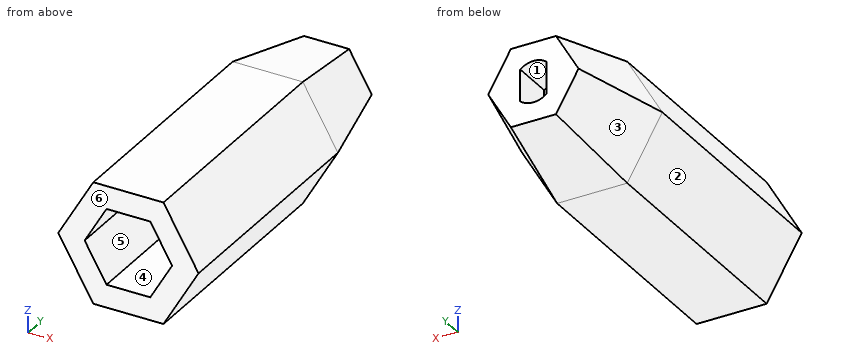
Autodesk Inventor part; units mm, degrees
ref_plane "YZ Plane" through (0, 0, 0) normal (1, 0, 0) x (0, 1, 0)
ref_plane "XZ Plane" through (0, 0, 0) normal (0, 1, 0) x (-1, 0, 0)
ref_plane "XY Plane" through (0, 0, 0) normal (0, 0, 1) x (1, 0, 0)
sketch "Boceto1" plane through (0, 0, 0) normal (0, 1, 0) x (-1, 0, 0)
  line L0 (0, 0) -> (5.8, 0)
  line L1 (5.8, 0) -> (9.3, 0)
  line L2 (5.8, 0) -> (2.9, -5.0229)
  line L3 (2.9, -5.0229) -> (-2.9, -5.0229)
  line L4 (-2.9, -5.0229) -> (-5.8, 0)
  line L5 (-5.8, 0) -> (-2.9, 5.0229)
  line L6 (-2.9, 5.0229) -> (2.9, 5.0229)
  line L7 (2.9, 5.0229) -> (5.8, 0)
  line L8 (9.3, 0) -> (4.65, -8.054)
  line L9 (4.65, -8.054) -> (-4.65, -8.054)
  line L10 (-4.65, -8.054) -> (-9.3, 0)
  line L11 (-9.3, 0) -> (-4.65, 8.054)
  line L12 (-4.65, 8.054) -> (4.65, 8.054)
  line L13 (4.65, 8.054) -> (9.3, 0)
  dimension "d0" = 5.8
  dimension "d1" = 3.5
extrude "Extrusión1" add sketch "Boceto1" along normal blind 30
sketch "Boceto2" plane through (0, 30, 0) normal (0, 1, 0) x (1, 0, 0)
  line L0 (-4.65, 8.054) -> (-9.3, 0)
  line L1 (-9.3, 0) -> (-4.65, 8.054)
  line L2 (-4.65, 8.054) -> (4.65, 8.054)
  line L3 (4.65, 8.054) -> (9.3, 0)
  line L4 (9.3, 0) -> (4.65, -8.054)
  line L5 (4.65, -8.054) -> (-4.65, -8.054)
  line L6 (-4.65, -8.054) -> (-9.3, 0)
  point P0 (0, 0)
  point P1 (0, 0)
extrude "Extrusión2" add sketch "Boceto2" along normal blind 13.5 draft -12
sketch "Boceto3" plane through (0, 0, 0) normal (0, -1, 0) x (1, 0, 0)
  line L0 (9.3, 0) -> (5.9866, 0)
  line L1 (9.3, 0) -> (4.65, -8.054)
  line L2 (4.65, -8.054) -> (-4.65, -8.054)
  line L3 (-4.65, -8.054) -> (-9.3, 0)
  line L4 (-9.3, 0) -> (-4.65, 8.054)
  line L5 (-4.65, 8.054) -> (4.65, 8.054)
  line L6 (4.65, 8.054) -> (9.3, 0)
  point P0 (0, 0)
  point P1 (0, 0)
sketch "Boceto4" plane through (0, 0, 0) normal (0, -1, 0) x (1, 0, 0)
  line L0 (5.8, 0) -> (2.9, -5.0229)
  line L1 (2.9, -5.0229) -> (-2.9, -5.0229)
  line L2 (-2.9, -5.0229) -> (-5.8, 0)
  line L3 (-5.8, 0) -> (-2.9, 5.0229)
  line L4 (-2.9, 5.0229) -> (2.9, 5.0229)
  line L5 (2.9, 5.0229) -> (5.8, 0)
  point P0 (0, 0)
  point P1 (0, 0)
extrude "Extrusión3" add sketch "Boceto3" along normal blind 2
sketch "Boceto5" plane through (0, -2, 0) normal (0, -1, 0) x (1, 0, 0)
  line L0 (0, 0) -> (5.8, 0)
  line L1 (5.8, 0) -> (2.9, -5.0229)
  line L2 (2.9, -5.0229) -> (-2.9, -5.0229)
  line L3 (-2.9, -5.0229) -> (-5.8, 0)
  line L4 (-5.8, 0) -> (-2.9, 5.0229)
  line L5 (-2.9, 5.0229) -> (2.9, 5.0229)
  line L6 (2.9, 5.0229) -> (5.8, 0)
  dimension "d8" = 5.8
extrude "Extrusión4" cut sketch "Boceto5" against normal blind 2
sketch "Boceto6" plane through (0, 43.5, 0) normal (0, 1, 0) x (1, 0, 0)
  line L0 (-1.75, 0) -> (-1.75, 2.1213)
  line L1 (-1.75, 0) -> (-1.75, -2.1213)
  line L2 (1.75, 0) -> (1.75, 2.1213)
  line L3 (1.75, 0) -> (1.75, -2.1213)
  arc A0 (-1.75, -2.1213) -> (1.75, -2.1213) centre (0, 0) ccw
  arc A1 (1.75, 2.1213) -> (-1.75, 2.1213) centre (0, 0) ccw
extrude "Extrusión5" cut sketch "Boceto6" against normal blind 5.5
properties part number "acopladorV3"
Design review of the part built by this model. Coordinates are the model's own, in mm. Face numbers are marked on the shaded views. A direction names the side the tool comes from. Round coordinates to 2 decimals unless told otherwise and drop trailing zeros. Write each loop counter-clockwise with the first axis right and the second up, starting at its lowest first coordinate (ties: lowest second). Pieces come first, ordered by that corner, then holes. Notation, with made-up numbers: (-32.75, -4) -> (11.25, -4) arc R30 ccw to (11.25, 18) -> close; hole circle Ø8 at (-32, 22.5). An arc over 180 degrees is marked (long way). Write item = value, one per line. Start each with the question number.
1) Wall thickness on probe 1 along Z at (x, y) = (-2, 0); probe 2 along X at (y, z) = (4.5, -0.5); probe 3 along Y at (x, z) = (0.75, -1.25): over which ranges is each line inside the solid? List them lowest first. Write a range as from..to.
2) Take a section at D-D, the plane x = 3.75. State the section outline as (y, z) points.
3) Take a section at C-C, the plane z = 1.25. State the section outline as (x, y) points.
4) Take a section at B-B, the plane x = 0. State the section outline as (y, z) points, plus the area to 3 significant figures.
5) Clearance check with flat-ended pins moving along their axes: pin 1 (3.5 mm diameter, centred on y = 41, z = 0, fed in from +X); pin 2 (8 mm diameter, centred on y = 32.5, z = 6, fed in from -X); pin 3 (6 mm diameter, centred on x = -7.5, y = 34, fed in from +Z). State where each tip first meets the part, or that it passes through.
6) Take a section at A-A, the plane y = 12. State the section outline as (x, z) points, plus the area to 3 significant figures.
7) Tool access review of the marked faces 1 and 2: name each direction out of +Z, -Z, +X, -X, +Y, -Y from which nothing blocks a thin tool from reaching the whole face with its end or side.
8) Mouldability with a two-part tool opening along Z and no side actions: class the marked faces 3, 4, 5 and 6 as +Z half, -Z half, draft (parallel to the pull), parting line (faces both ways), or undercut.
Results list:
q1.probe_1 = -8.05..-5.02, 5.02..8.05
q1.probe_2 = -9.01..-5.51, 5.51..9.01
q1.probe_3 = 30..38
q2.outline = (-2, -8.05) -> (30, -8.05) -> (37.33, -6.5) -> (43.5, -3.87) -> (43.5, 3.87) -> (37.33, 6.5) -> (30, 8.05) -> (-2, 8.05) -> (-2, 3.55) -> (30, 3.55) -> (30, -3.55) -> (-2, -3.55) -> close
q3.outline = (-8.58, -2) -> (-5.08, -2) -> (-5.08, 30) -> (5.08, 30) -> (5.08, -2) -> (8.58, -2) -> (8.58, 30) -> (5.26, 43.5) -> (1.75, 43.5) -> (1.75, 38) -> (-1.75, 38) -> (-1.75, 43.5) -> (-5.26, 43.5) -> (-8.58, 30) -> close
q4.outline = (-2, -8.05) -> (30, -8.05) -> (43.5, -5.18) -> (43.5, -2.75) -> (38, -2.75) -> (38, 2.75) -> (43.5, 2.75) -> (43.5, 5.18) -> (30, 8.05) -> (-2, 8.05) -> (-2, 5.02) -> (30, 5.02) -> (30, -5.02) -> (-2, -5.02) -> close
q4.area = 342 mm²
q5.pin_1 = 7.03
q5.pin_2 = -7.73
q5.pin_3 = 6.77
q6.outline = (-9.3, 0) -> (-4.65, -8.05) -> (4.65, -8.05) -> (9.3, 0) -> (4.65, 8.05) -> (-4.65, 8.05) -> close; hole (-5.8, 0) -> (-2.9, -5.02) -> (2.9, -5.02) -> (5.8, 0) -> (2.9, 5.02) -> (-2.9, 5.02) -> close
q6.area = 137 mm²
q7.face_1 = +Y
q7.face_2 = -Z, -X, +Y, -Y
q8.face_3 = -Z half
q8.face_4 = undercut
q8.face_5 = undercut
q8.face_6 = draft
